Could you check a few things on this model? Use its own coordinates, in mm. Face numbers are marked on the shaded views. A direction names the side the tool comes from. Round coordinates to 2 decimals unless told otherwise and drop trailing zeros. Order: outer loops, then holes, each group sorted by start corner. A loop starts at its lowest first (then second) coordinate and runs counter-clockwise, first axis right, second up.
```python
from build123d import *

# Parameters (mm, degrees)
BOSS_EXTRUDE1_DEPTH    = 370
CUT_EXTRUDE1_REACH     = 376.267
SKETCH4_R              = 5
CUT_EXTRUDE2_DEPTH     = 375.566416007
SKETCH5_R              = 2.5
CUT_EXTRUDE3_DEPTH     = 375.566416007
SKETCH6_R              = 2.5
CUT_EXTRUDE4_DEPTH     = 375.566416007
CONVERT_SOLID1_DEPTH   = 370
CONVERT_SOLID1_2_DEPTH = 370
FILLET1_R              = 4


# Read off the part's stored shape, not the designer's step: Convert-Solid1
with BuildPart() as part:
    # Sketch1 → Boss-Extrude1 (new body)
    with BuildSketch(Plane.XY):
        Polygon((0, 0), (0, 4), (26, 4), (26, 50), (30, 50), (30, 0), align=None)
    extrude(amount=BOSS_EXTRUDE1_DEPTH)

    # Sketch3 → Cut-Extrude1 (cut, up to next)
    with BuildSketch(Plane.ZY.offset(-26), mode=Mode.PRIVATE) as cut_extrude1_sk1:
        with BuildLine():
            Line((150, 35), (290, 35))
            ThreePointArc((290, 35), (295, 30), (290, 25))
            Line((290, 25), (150, 25))
            ThreePointArc((150, 25), (145, 30), (150, 35))
        make_face()
    cut_extrude1_tool1 = extrude(cut_extrude1_sk1.sketch, amount=-CUT_EXTRUDE1_REACH, mode=Mode.PRIVATE) & part.part
    add(cut_extrude1_tool1.solids().sort_by_distance((26, 30, 220))[0], mode=Mode.SUBTRACT)

    # Sketch4 → Cut-Extrude2 (cut, through all)
    with BuildSketch(Plane(origin=(30, 0, 0), x_dir=(0, 0, -1), z_dir=(1, 0, 0))):
        with Locations(Location((-48, 30, 0), (0, 0, 90))):
            Circle(SKETCH4_R)
    extrude(amount=-CUT_EXTRUDE2_DEPTH, mode=Mode.SUBTRACT)

    # Sketch5 → Cut-Extrude3 (cut, through all)
    with BuildSketch(Plane.XZ):
        with Locations((8.2, 27.7)):
            Circle(SKETCH5_R)
    extrude(amount=-CUT_EXTRUDE3_DEPTH, mode=Mode.SUBTRACT)

    # Sketch6 → Cut-Extrude4 (cut, through all)
    with BuildSketch(Plane.XZ):
        with Locations((8.2, 342.3)):
            Circle(SKETCH6_R)
    extrude(amount=-CUT_EXTRUDE4_DEPTH, mode=Mode.SUBTRACT)

    # Convert-Solid1 outline → Convert-Solid1 (cut)
    with BuildSketch(Plane.XY):
        with BuildLine():
            ThreePointArc((30, 8), (27.656854249, 2.343145751), (22, 0))
            Line((22, 0), (30, 0))
            Line((30, 0), (30, 8))
        make_face()
    extrude(amount=CONVERT_SOLID1_DEPTH, mode=Mode.SUBTRACT)

    # Convert-Solid1 2 outline → Convert-Solid1 2 (add)
    with BuildSketch(Plane.XY):
        with BuildLine():
            ThreePointArc((26, 8), (24.828427125, 5.171572875), (22, 4))
            Line((22, 4), (26, 4))
            Line((26, 4), (26, 8))
        make_face()
    extrude(amount=CONVERT_SOLID1_2_DEPTH)

    # Fillet1
    fillet1_edges = [part.edges().sort_by_distance(p)[0] for p in [
        (28, 50, 0),
        (28, 50, 370),
        (0, 2, 370),
        (0, 2, 0),
    ]]
    fillet(fillet1_edges, radius=FILLET1_R)


solid = part.part
```
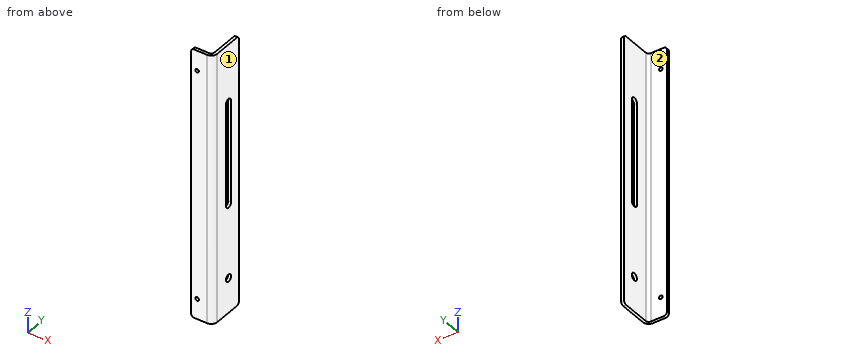
Q1. Imagine slicing it at A-A, the plane y = 30. Please give me the cut outline in (x, z), then the cut area to 3 significant figures.
Q2. For the marked faces 1 and 2, which set-ups out of +Z, -Z, +X, -X, +Y, -Y let a thin tool reach every point of the face, with its end or its side?
Q3. For P1, Ø3, axis at x = 28.5, z = 238.5, coming from the -Y side (3 decimals); P2, Ø4, axis at y = 38, z = 68, coming from the -X side; P3, Ø6.5, axis at x = 11, z = 170.5, coming from the +Y side, each with a flat end and sliding along its axis, tell me the tip position at first contact or that it passes through.
Q4. Imagine slicing it at B-B, the plane z = 218. Please give me the cut outline in (x, y), then the cut area to 3 significant figures.
Q5. I need wall thicknesses on L1, parallel to Z at x = 29.1, y = 30; L2, parallel to Z at x = 8.2, y = 2.7; L3, parallel to Y at x = 21, z = 67. Which ranges of each line are inside material? Lowest first, please.
Filled in:
1. outline: (26, 0) - (30, 0) - (30, 43) - (26, 43) - close; (26, 53) - (30, 53) - (30, 145) - (26, 145) - close; (26, 295) - (30, 295) - (30, 370) - (26, 370) - close
1. area: 840 mm2
2. face 1: +Z, -Z, +X, +Y, -Y
2. face 2: +Z, -Z, -X, +Y
3. P1: stops at y = 1.755
3. P2: stops at x = 26
3. P3: stops at y = 4
4. outline: (0, 0) - (22, 0) arc R8 ccw to (30, 8) - (30, 25) - (26, 25) - (26, 8) arc R4 cw to (22, 4) - (0, 4) - close; (26, 35) - (30, 35) - (30, 50) - (26, 50) - close
4. area: 254 mm2
5. L1: z = 0 to 43, 53 to 145, 295 to 370
5. L2: z = 0 to 25.2, 30.2 to 339.8, 344.8 to 370
5. L3: y = 0 to 4
